```python
from build123d import *

# Parameters (mm, degrees)
SKETCH6_R           = 3
SKETCH6_W           = 6.2
SKETCH6_H           = 6.2
BOSS_EXTRUDE4_DEPTH = 6.2
CUT_EXTRUDE3_DEPTH  = 1


with BuildPart() as part:
    # Sketch6 → Boss-Extrude4 (new body)
    with BuildSketch(Plane.XY):
        Polygon((157.908027241, 124.653899243), (153.794027241, 124.653899243), (153.794027241, 37.653899243), (132.344027241, 37.653899243), (132.344027241, 31.453899243), (126.144027241, 31.453899243), (126.144027241, 37.653899243), (119.944027241, 37.653899243), (119.944027241, 31.453899243), (113.744027241, 31.453899243), (113.744027241, 37.653899243), (107.544027241, 37.653899243), (107.544027241, -5.346100757), (182.594027241, -5.346100757), (182.594027241, 7.653899243), (188.794027241, 7.653899243), (188.794027241, 20.653899243), (182.594027241, 20.653899243), (182.594027241, 31.453899243), (176.394027241, 31.453899243), (176.394027241, 37.653899243), (182.594027241, 37.653899243), (182.594027241, 33.653899243), (188.794027241, 33.653899243), (188.794027241, 46.653899243), (182.594027241, 46.653899243), (182.594027241, 59.653899243), (188.794027241, 59.653899243), (188.794027241, 72.653899243), (182.594027241, 72.653899243), (182.594027241, 85.653899243), (188.794027241, 85.653899243), (188.794027241, 98.653899243), (182.594027241, 98.653899243), (182.594027241, 111.653899243), (188.794027241, 111.653899243), (188.794027241, 124.653899243), (178.478027241, 124.653899243), (178.478027241, 118.453899243), (174.364027241, 118.453899243), (174.364027241, 124.653899243), (170.250027241, 124.653899243), (170.250027241, 118.453899243), (166.136027241, 118.453899243), (166.136027241, 124.653899243), (162.022027241, 124.653899243), (162.022027241, 118.453899243), (157.908027241, 118.453899243), align=None)
        with Locations((123.115137004, 25.259504391)):
            Circle(SKETCH6_R, mode=Mode.SUBTRACT)
        with Locations((167.094027241, 34.553899243)):
            Rectangle(SKETCH6_W, SKETCH6_H, mode=Mode.SUBTRACT)
    extrude(amount=BOSS_EXTRUDE4_DEPTH)

    # Sketch7 → Cut-Extrude3 (cut)
    with BuildSketch(Plane.XY.offset(6.2)):
        with BuildLine():
            Line((115.946331614, 11.576783669), (115.946331614, 11.251142644))
            Line((115.946331614, 11.251142644), (114.866373682, 11.251142644))
            Line((114.866373682, 11.251142644), (114.69528494, 10.416051498))
            add(Edge.make_bspline(
                [(114.69528494, 10.416051498), (114.728899911, 10.425331816), (114.794023603, 10.443310964), (114.890144334, 10.463273342), (114.981395832, 10.475306994), (115.040609919, 10.476950112), (115.069263305, 10.477745208)],
                knots=[0, 0, 0, 0, 0.000104595, 0.000202637, 0.000294305, 0.000380252, 0.000380252, 0.000380252, 0.000380252], degree=3))
            add(Edge.make_bspline(
                [(115.069263305, 10.477745208), (115.10471784, 10.476977823), (115.174430315, 10.475468954), (115.276428503, 10.460980204), (115.37379477, 10.43817471), (115.466325492, 10.40631538), (115.554191848, 10.365575836), (115.636585422, 10.314685176), (115.714742957, 10.255237083), (115.78726231, 10.186888393), (115.853052218, 10.111666641), (115.910897081, 10.030787715), (115.960030287, 9.945037622), (115.999546115, 9.853597069), (116.031100475, 9.75747698), (116.052102642, 9.655665995), (116.0660878, 9.549123772), (116.06765025, 9.476276054), (116.068446999, 9.439128421)],
                knots=[0, 0, 0, 0, 0.000106308, 0.000209029, 0.000308378, 0.000405929, 0.000502102, 0.000598312, 0.00069588, 0.000796219, 0.000896736, 0.000995218, 0.001094066, 0.001192613, 0.001293582, 0.001396995, 0.001504047, 0.001615439, 0.001615439, 0.001615439, 0.001615439], degree=3))
            add(Edge.make_bspline(
                [(116.068446999, 9.439128421), (116.067843681, 9.413254692), (116.066645197, 9.361856897), (116.060550479, 9.285526086), (116.048815936, 9.21081123), (116.033060929, 9.137702418), (116.012611736, 9.066338059), (115.987856666, 8.996513887), (115.957561698, 8.928664494), (115.924331807, 8.862147885), (115.886915359, 8.798467811), (115.845387713, 8.738914802), (115.801513304, 8.682595489), (115.754304332, 8.630113888), (115.703322001, 8.581814865), (115.649183746, 8.537411781), (115.592321565, 8.496153717), (115.531855738, 8.459715426), (115.469133628, 8.426184744), (115.40324946, 8.398676964), (115.335702967, 8.374083842), (115.265521973, 8.354480913), (115.192865443, 8.339120668), (115.117613611, 8.32868798), (115.040161146, 8.321089354), (114.987660242, 8.320613688), (114.961140308, 8.320373413)],
                knots=[0, 0, 0, 0, 7.7636e-05, 0.000154223, 0.000229512, 0.000304362, 0.000378447, 0.000452077, 0.000526407, 0.000601214, 0.00067506, 0.000747747, 0.00081887, 0.000889121, 0.000959302, 0.001029336, 0.001099058, 0.00116985, 0.001240974, 0.00131221, 0.00138383, 0.001456517, 0.001530612, 0.001606437, 0.001684346, 0.001763871, 0.001763871, 0.001763871, 0.001763871], degree=3))
            add(Edge.make_bspline(
                [(114.961140308, 8.320373413), (114.929504444, 8.321000102), (114.867264619, 8.322233038), (114.776078105, 8.335131235), (114.688344141, 8.353604216), (114.604768978, 8.38139569), (114.524603617, 8.41621845), (114.448927295, 8.460229548), (114.375806341, 8.51010345), (114.308213279, 8.568959198), (114.245478804, 8.633289853), (114.189320757, 8.703101427), (114.139306727, 8.777241707), (114.096237628, 8.856070747), (114.059500137, 8.939381414), (114.030639398, 9.02748585), (114.007345461, 9.119923711), (113.997490787, 9.183562967), (113.99248546, 9.215886233)],
                knots=[0, 0, 0, 0, 9.4843e-05, 0.000186593, 0.000275792, 0.000363484, 0.000450342, 0.000537514, 0.000625728, 0.000715478, 0.000805885, 0.000894984, 0.00098389, 0.001073836, 0.001164117, 0.001256635, 0.001351658, 0.001449737, 0.001449737, 0.001449737, 0.001449737], degree=3))
            Line((113.99248546, 9.215886233), (114.277421358, 9.215886233))
            add(Edge.make_bspline(
                [(114.277421358, 9.215886233), (114.284432264, 9.185609023), (114.297907613, 9.127414543), (114.327485686, 9.045652541), (114.36364973, 8.972791531), (114.406652246, 8.907867695), (114.457951202, 8.851253818), (114.516488613, 8.800801198), (114.582118333, 8.755285188), (114.655046477, 8.717345963), (114.731984056, 8.684989308), (114.812508596, 8.663443128), (114.894427539, 8.648293032), (114.949834347, 8.646776506), (114.977676767, 8.646014439)],
                knots=[0, 0, 0, 0, 9.3172e-05, 0.000179081, 0.000260145, 0.000336703, 0.000411917, 0.000488562, 0.000568128, 0.000650923, 0.00073478, 0.000817953, 0.000900557, 0.000983994, 0.000983994, 0.000983994, 0.000983994], degree=3))
            add(Edge.make_bspline(
                [(114.977676767, 8.646014439), (115.004853355, 8.646759001), (115.058364281, 8.648225052), (115.137114611, 8.659509013), (115.213144861, 8.676887667), (115.28570482, 8.702895321), (115.356064217, 8.734504458), (115.42244328, 8.77506742), (115.486762318, 8.821749008), (115.547022125, 8.875231094), (115.602212197, 8.934167888), (115.650976678, 8.997193809), (115.691595736, 9.064428377), (115.725825963, 9.134707595), (115.751818598, 9.208801714), (115.770361488, 9.286363495), (115.781249978, 9.367584512), (115.782747834, 9.4229831), (115.783511101, 9.451212756)],
                knots=[0, 0, 0, 0, 8.15e-05, 0.000160473, 0.000238226, 0.000315066, 0.000391338, 0.000469218, 0.000547964, 0.000629516, 0.000710512, 0.000789892, 0.000868102, 0.000945761, 0.001024012, 0.00110315, 0.001184644, 0.001269321, 0.001269321, 0.001269321, 0.001269321], degree=3))
            add(Edge.make_bspline(
                [(115.783511101, 9.451212756), (115.782913767, 9.476681473), (115.781744568, 9.526532864), (115.772191837, 9.59946643), (115.755575726, 9.668475547), (115.732512635, 9.733893459), (115.70323051, 9.795781868), (115.66744707, 9.854204644), (115.624490773, 9.908391764), (115.575421703, 9.95836858), (115.521666194, 10.004492145), (115.46229937, 10.043811424), (115.39856358, 10.076889406), (115.331226729, 10.105435376), (115.258687142, 10.125937481), (115.18238134, 10.141329777), (115.101485326, 10.150233713), (115.046176202, 10.15146914), (115.017745877, 10.152104182)],
                knots=[0, 0, 0, 0, 7.6388e-05, 0.000149519, 0.000220172, 0.000288967, 0.000357247, 0.000425206, 0.000494043, 0.000564207, 0.000635056, 0.000706145, 0.000777268, 0.000850264, 0.000925136, 0.001002969, 0.001083601, 0.001168886, 0.001168886, 0.001168886, 0.001168886], degree=3))
            add(Edge.make_bspline(
                [(115.017745877, 10.152104182), (114.993136063, 10.151577503), (114.942323041, 10.150490044), (114.864378762, 10.142483151), (114.782471271, 10.129566076), (114.69691455, 10.111798552), (114.60745166, 10.088547504), (114.514271397, 10.060685064), (114.417177841, 10.027372965), (114.351756762, 10.002215885), (114.318126486, 9.989283669)],
                knots=[0, 0, 0, 0, 7.3822e-05, 0.000152423, 0.000234822, 0.000322511, 0.00041445, 0.000512043, 0.000614219, 0.000722306, 0.000722306, 0.000722306, 0.000722306], degree=3))
            Line((114.318126486, 9.989283669), (114.643767512, 11.576783669))
            Line((114.643767512, 11.576783669), (115.946331614, 11.576783669))
        make_face()
        Polygon((118.127236061, 11.658193926), (118.185113666, 11.658193926), (118.185113666, 9.460117003), (118.551459819, 9.460117003), (118.551459819, 9.134475977), (118.185113666, 9.134475977), (118.185113666, 8.401783669), (117.900177768, 8.401783669), (117.900177768, 9.134475977), (116.394088025, 9.134475977), align=None)
        Polygon((117.900177768, 9.460117003), (117.900177768, 10.839003221), (116.953783537, 9.460117003), align=None, mode=Mode.SUBTRACT)
    extrude(amount=-CUT_EXTRUDE3_DEPTH, mode=Mode.SUBTRACT)


solid = part.part
```
CAD build for the part. Positions are in the model's coordinates, mm. A direction names the side the tool comes from. Round coordinates to 2 decimals unless told otherwise and drop trailing zeros. Write each loop counter-clockwise with the first axis right and the second up, starting at its lowest first coordinate (ties: lowest second). Pieces come first, ordered by that corner, then holes. Notation, with made-up numbers: (46.25, 32) -> (98.25, 32) arc R29 ccw to (98.25, 53) -> close; hole circle Ø11 at (76.25, -2.75). An arc over 180 degrees is marked (long way). Answer in a Markdown table with one row per item. Add a question column.
Item 1: Saw through at A-A, the plane x = 122. Write the cut outline in (y, z), then the cut area to 3 significant figures.
Item 2: Drop flat-ended pins along their axis: pin 1 Ø1.9 at (x, z) = (112, 2.5) entering from +Y; pin 2 Ø1.5 at (x, z) = (129, 4) entering from +Y; pin 3 Ø1.9 at (x, z) = (187, 2) entering from -Y. Give the stop position or say it passes through.
Item 3: Drill centre lines: line 1 (Y direction, x = 168.5, z = 2.5); line 2 (X direction, y = 33, z = 4.75); line 3 (X direction, y = 96, z = 5.75). Where is each one in solid material? Low to high. Write a range as from..to.
Item 4: Which spindle directions (+Z, -Z, +X, -X, +Y, -Y) get a long thin tool onto all of the face, cutting with end or side? Do faces 4 (the face through (111, 37.654, 3)), 5 (the face through (186, 7.654, 3)), 6 (the face through (119.944, 35, 3)), 7 (the face through (186, 111.654, 3)). Say none if no direction does.
Item 5: Saw through at D-D, the plane z = 3.25. Count the separate pieces of the cut face and the enclosed holes in it, then the cut area to 3 significant figures.
Item 6: Saw through at B-B, the plane y = 57.5. Write the cut outline in (x, z).
Item 7: Saw through at C-C, the plane x = 160.5. Write the cut outline in (y, z).
Item 8: Mould opens along X. For faces 1 (the face through (186, 72.654, 3)), 2 (the face through (188.794, 40, 3)), 3 (the face through (170.194, 35, 3)) say: pulls with the +X half, pulls with the -X half, needs draft (parallel to the pull), parting line crosses it, or undercut.
Findings below:
| question | item | result |
|---|---|---|
| 1 | outline | (-5.35, 0) -> (22.47, 0) -> (22.47, 6.2) -> (-5.35, 6.2) -> close; (28.04, 0) -> (37.65, 0) -> (37.65, 6.2) -> (28.04, 6.2) -> close |
| 1 | area | 232 mm^2 |
| 2 | pin 1 | stops at y = 37.65 |
| 2 | pin 2 | stops at y = 31.45 |
| 2 | pin 3 | stops at y = 7.65 |
| 3 | line 1 | y = -5.35..31.45, 37.65..118.45 |
| 3 | line 2 | x = 107.54..113.74, 119.94..126.14, 132.34..163.99, 170.19..176.39 |
| 3 | line 3 | x = 153.79..188.79 |
| 4 | face 4 | +Z, -Z, -X, +Y |
| 4 | face 5 | +Z, -Z, +X, -Y |
| 4 | face 6 | +Z, -Z, +Y |
| 4 | face 7 | +Z, -Z, +X |
| 5 | separate pieces | 1 |
| 5 | enclosed holes | 2 |
| 5 | area | 5,880 mm^2 |
| 6 | outline | (153.79, 0) -> (182.59, 0) -> (182.59, 6.2) -> (153.79, 6.2) -> close |
| 7 | outline | (-5.35, 0) -> (118.45, 0) -> (118.45, 6.2) -> (-5.35, 6.2) -> close |
| 8 | face 1 | needs draft |
| 8 | face 2 | pulls with the +X half |
| 8 | face 3 | undercut |
